Source: CAD feature listing. Evaluate the final solid. Frame: model axes, mm. A direction names the side the tool comes from. Give positions to 0.01 mm unless a question says otherwise; leave off trailing zeros. Write each loop counter-clockwise with the first axis right and the second up, starting at its lowest first coordinate (ties: lowest second). Pieces come first, ordered by that corner, then holes. Notation, with made-up numbers: (-12.5, -0.5) -> (0.5, -0.5) arc R34 cw to (0.5, 32.5) -> close; hole circle Ø11 at (-4, 52.25). An arc over 180 degrees is marked (long way). Write item = value, one per line.
from build123d import *

# Parameters (mm, degrees)
SKETCH1_R           = 2.1
BOSS_EXTRUDE1_DEPTH = 10
FILLET1_R           = 1


with BuildPart() as part:
    # Sketch1 → Boss-Extrude1 (new body)
    with BuildSketch(Plane.XY):
        Polygon((3, 10), (3, 8), (6, 8), (2, 4), (-2, 4), (-6, 8), (-3, 8), (-3, 10), (-10, 10), (-10, 3), (-8, 3), (-8, 6), (-4, 2), (-4, -2), (-8, -6), (-8, -3), (-10, -3), (-10, -10), (-3, -10), (-3, -8), (-6, -8), (-2, -4), (2, -4), (6, -8), (3, -8), (3, -10), (10, -10), (10, -3), (8, -3), (8, -6), (4, -2), (4, 2), (8, 6), (8, 3), (10, 3), (10, 10), align=None)
        Circle(SKETCH1_R, mode=Mode.SUBTRACT)
    extrude(amount=BOSS_EXTRUDE1_DEPTH)

    # Fillet1
    fillet1_edges = [part.edges().sort_by_distance(p)[0] for p in [
        (-10, 10, 5),
        (10, 10, 5),
        (10, -10, 5),
        (-10, -10, 5),
    ]]
    fillet(fillet1_edges, radius=FILLET1_R)


solid = part.part
(1) Section query B-B (y = 3.25). Return loops of the section in (x, z).
Values follow:
outline = (-10, 0) -> (-8, 0) -> (-8, 10) -> (-10, 10) -> close; (-5.25, 0) -> (5.25, 0) -> (5.25, 10) -> (-5.25, 10) -> close; (8, 0) -> (10, 0) -> (10, 10) -> (8, 10) -> close
(2) First-contact query: pin 1 (2 mm diameter, centred on y = -9.5, z = 4, fed in from +X); pin 2 (4.5 mm diameter, centred on y = -0.5, z = 5.5, fed in from -X); pin 3 (1 mm diameter, centred on x = -7, y = 3, fed in from -Z); pin 4 (3 mm diameter, centred on x = 1, z = 5, fed in from -Y). Flat tips, straight axial feed; report the tip coordinate or a pass-through.
Values follow:
pin_1 = 10
pin_2 = -4.75
pin_3 = through
pin_4 = -4.5
(3) Section query D-D (y = 0). Return loops of the section in (x, z).
Values follow:
outline = (-4, 0) -> (-2.1, 0) -> (-2.1, 10) -> (-4, 10) -> close; (2.1, 0) -> (4, 0) -> (4, 10) -> (2.1, 10) -> close
(4) Pull-direction query (Y, two-part tool) for faces 1 (the face through (-4, 6, 5)), 2 (the face through (0, 4, 5)), 3 (the face through (-3, 9, 5)), 4 (the face through (-4, -8, 5)); classes: pulls with the +Y half, pulls with the -Y half, needs draft (parallel to the pull), parting line crosses it, or undercut.
Values follow:
face_1 = undercut
face_2 = pulls with the +Y half
face_3 = needs draft
face_4 = undercut
(5) Access query for faces 5 (the face through (3, 9, 5)), 6 (the face through (9.715, -9.699, 5.07)), 7 (the face through (4, -6, 5)), 8 (the face through (3, -9, 5)), 9 (the face through (-4, 0, 5)). Directions: +Z, -Z, +X, -X, +Y, -Y. A direction counts if a zero-diameter tool reaches every point of the face in a straight line with its end or side. Return the directions, or none.
Values follow:
face_5 = +Z, -Z, +Y
face_6 = +Z, -Z, +X, -Y
face_7 = +Z, -Z
face_8 = +Z, -Z, -Y
face_9 = +Z, -Z, -X
(6) Section query A-A (x = -7.75). Return loops of the section in (y, z).
Values follow:
outline = (-10, 0) -> (-5.75, 0) -> (-5.75, 10) -> (-10, 10) -> close; (5.75, 0) -> (10, 0) -> (10, 10) -> (5.75, 10) -> close
(7) Section query C-C (x = -3.75). Return loops of the section in (y, z), plus the area to 3 significant figures.
Values follow:
outline = (-10, 0) -> (-8, 0) -> (-8, 10) -> (-10, 10) -> close; (-5.75, 0) -> (5.75, 0) -> (5.75, 10) -> (-5.75, 10) -> close; (8, 0) -> (10, 0) -> (10, 10) -> (8, 10) -> close
area = 155 mm2
(8) Material intervals for line 1 (Y direction, x = 0, z = 4.75); line 2 (X direction, y = 5.5, z = 6); line 3 (X direction, y = 8.75, z = 1), sorted ascending.
Values follow:
line_1 = -4 to -2.1, 2.1 to 4
line_2 = -10 to -8, -7.5 to -3.5, 3.5 to 7.5, 8 to 10
line_3 = -10 to -3, 3 to 10
